from build123d import *

# Parameters (mm, degrees)
F0_R            = 63.5
F0_R_2          = 14.4272
F1_DEPTH        = 3.175
F2_W            = 12.7
F2_H            = 6.35
F3_DEPTH        = 3.176
F3_COPIES_COUNT = 12
F4_R            = 2.4892
F5_DEPTH        = 182


# Not quite as in the source:
# - an extrude ends at something that could not be found from the text; its depth is read off the source's solid
# - a pattern or mirror of a feature is missing from the dataset's text; its kind, count and spacing are read off the source's solid


with BuildPart() as f1:
    # F0 (on Top) → F1 (new body)
    with BuildSketch(Plane.XY):
        Circle(F0_R)
        Circle(F0_R_2, mode=Mode.SUBTRACT)
    extrude(amount=F1_DEPTH)

    # F2 (on face) → F3 (cut, through all)
    with BuildSketch(Plane.XY.offset(3.175)):
        with Locations((0, 43.815)):
            Rectangle(F2_W, F2_H)
    f3 = extrude(amount=-F3_DEPTH, mode=Mode.SUBTRACT)

    # F3_copies: F3 ×12 about axis
    f3_copies_axis = Axis((0, 0, 0), (0, 0, 1))
    for i in range(1, F3_COPIES_COUNT):
        add(f3.rotate(f3_copies_axis, i * 360 / F3_COPIES_COUNT), mode=Mode.SUBTRACT)

    # F4 (on Top) → F5 (cut, through all)
    with BuildSketch(Plane.XY):
        with Locations((0, 23.8125)):
            Circle(F4_R)
    extrude(amount=-F5_DEPTH, mode=Mode.SUBTRACT)


solid = f1.part
Verification items for the finished model (mm, model axes). Give positions to 0.01 mm unless a question says otherwise; leave off trailing zeros. Write each loop counter-clockwise with the first axis right and the second up, starting at its lowest first coordinate (ties: lowest second). Pieces come first, ordered by that corner, then holes. Notation, with made-up numbers: M 35.5,64 L 66.5,64 A19 cw 66.5,88 Z; hole C 24.25,31.5 d2. An arc over 180 degrees is marked long. Put each result on its own line as item: value. Start each with the question number.
1. Scan lines: line 1 along Y through (x, z) = (0, 1); line 2 along X through (y, z) = (-37, 1.85); line 3 along X through (y, z) = (19.5, 1.35). Record each from-to range of solid material in increasing order. Write a range as [from, to].
2. Section check D-D (z = 1.8). Give the number of separate pieces and of enclosed holes in the cut face, and give its area (3 significant figures).
3. Go/stop test with flat-tipped pins: pin 1 Ø1 at (y, z) = (-44.5, 1.5) entering from -X; pin 2 Ø1.5 at (y, z) = (-44.5, 0.5) entering from -X; pin 3 Ø1.5 at (x, z) = (11.5, 2.5) entering from +Y. Record where each tip stops, or that it passes through.
4. Section check A-A (x = 0). Record the cut outline in (y, z) (3 decimals), and give its area (3 significant figures).
5. Section check C-C (x = -19.5). Record the cut outline in (y, z) (3 decimals).
6. Draft check along Y on faces 1 (the face through (20.4, -35.15, 1.61)), 2 (the face through (23.42, 40.74, 1.61)), 3 (the face through (-13.77, -61.99, 1.57)). Enter one of: +Y half, -Y half, draft (parallel to the pull), parting line (faces both ways), or undercut.
Answer list:
1. line 1: [-63.5, -46.99], [-40.64, -14.43], [14.43, 40.64], [46.99, 63.5]
1. line 2: [-51.61, -28.69], [-17.19, 17.19], [28.69, 51.61]
1. line 3: [-60.43, -43], [-35.67, 35.67], [43, 60.43]
2. separate pieces: 1
2. enclosed holes: 13
2. area: 11,000 mm2
3. pin 1: x = -45.78
3. pin 2: x = -46.02
3. pin 3: y = 62.58
4. outline: M -63.5,0 L -46.99,0 L -46.99,3.175 L -63.5,3.175 Z; M -40.64,0 L -14.427,0 L -14.427,3.175 L -40.64,3.175 Z; M 14.427,0 L 40.64,0 L 40.64,3.175 L 14.427,3.175 Z; M 46.99,0 L 63.5,0 L 63.5,3.175 L 46.99,3.175 Z
4. area: 271 mm2
5. outline: M -60.432,0 L -43.001,0 L -43.001,3.175 L -60.432,3.175 Z; M -35.669,0 L 35.669,0 L 35.669,3.175 L -35.669,3.175 Z; M 43.001,0 L 60.432,0 L 60.432,3.175 L 43.001,3.175 Z
6. face 1: undercut
6. face 2: undercut
6. face 3: parting line
